Read the model definition and answer for the solid it produces. Units are mm, in the model's axes. Face numbers are marked on the shaded views. A direction names the side the tool comes from. Coordinates: 2 decimals unless noted, no trailing zeros. Write each loop counter-clockwise with the first axis right and the second up, starting at its lowest first coordinate (ties: lowest second). Pieces come first, ordered by that corner, then holes.
Item 1: Section D-D (z = -31) is taken. Give the vertices of the cut face in (x, y), then the cut area to 3 significant figures.
Item 2: A tool of negligible diameter and unlimited length cuts with its end or side. For the marked faces 1, 2, 3 and 4, from which of +Z, -Z, +X, -X, +Y, -Y can it reach the whole face along a straight path? Write none if from no direction.
Item 3: Straight lines are drawn through the part: probe 1 along Y at (x, z) = (-27, -81); probe 2 along Z at (x, y) = (-8.5, 10); probe 3 along Z at (x, y) = (-8.5, 41.5). For each, find the intervals that lie inside material, in ascending order.
Item 4: Section C-C (y = 25) is taken. Give the vertices of the cut face in (x, z).
Item 5: Each of these flat-tipped pins is pushed along its axis until it touches: P1, Ø1.5, axis at y = 23.5, z = -97.5, coming from the +X side; P2, Ø8, axis at x = -10, z = -58, coming from the +Y side; P3, Ø2, axis at x = -4.5, z = 14, coming from the -Y side. Where does it stop, or does it pass through?
Item 6: Section A-A (x = -8.5) is taken. Give the vertices of the cut face in (y, z).
Item 7: Determine the mould class of the marked faces 5, 6 and 7 for opening direction Z: released by +Z, released by -Z, zero draft, split by the parting line, or undercut.
Item 8: Section B-B (z = -81) is taken. Give the vertices of the cut face in (x, y), then the cut area to 3 significant figures.
Autodesk Inventor part; units mm, degrees
ref_plane "YZ Plane" through (0, 0, 0) normal (1, 0, 0) x (0, 1, 0)
ref_plane "XZ Plane" through (0, 0, 0) normal (0, 1, 0) x (-1, 0, 0)
ref_plane "XY Plane" through (0, 0, 0) normal (0, 0, 1) x (1, 0, 0)
sketch "Sketch1" plane through (0, 0, 0) normal (0, 1, 0) x (-1, 0, 0)
  arc A0 (35, -5) -> (0, 30) centre (0, -5) ccw
  line L0 (34.641, 0) -> (0, 0)
  line L1 (-35, -5) -> (-35, -100) construction
  line L2 (-35, -100) -> (0, -100) construction
  line L3 (35, -100) -> (35, -5)
  line L4 (0, -100) -> (0, 30)
  arc A1 (0, 30) -> (-35, -5) centre (0, -5) ccw construction
  line L5 (0, -5) -> (-35, -5) construction
  line L6 (0, -100) -> (35, -100)
  dimension "d0" = 70
  dimension "d1" = 130
  dimension "d32" = 30
  dimension "d33" = 35
  dimension "d34" = 5
extrude "Extrusion1" add sketch "Sketch1" along normal blind 50
sketch "Sketch2" plane through (0, 0, 30) normal (1, 0, 0) x (0, 0, -1)
  line L0 (19, 49) -> (27.5, 49)
  line L1 (59, 49) -> (59, 40)
  line L2 (59, 9) -> (19, 9)
  line L3 (19, 9) -> (19, 14)
  line L4 (19, 40) -> (12, 40)
  line L5 (12, 40) -> (12, 37)
  line L6 (12, 37) -> (19, 37)
  line L7 (19, 37) -> (19, 40) construction
  line L8 (19, 17) -> (14, 17)
  line L9 (14, 17) -> (14, 14)
  line L10 (14, 14) -> (19, 14)
  line L11 (19, 14) -> (19, 17) construction
  line L12 (59, 40) -> (66, 40)
  line L13 (66, 40) -> (66, 37)
  line L14 (66, 37) -> (59, 37)
  line L15 (59, 37) -> (59, 40) construction
  line L16 (27.5, 49) -> (32.5, 49) construction
  line L17 (32.5, 49) -> (32.5, 54)
  line L18 (32.5, 54) -> (27.5, 54)
  line L19 (27.5, 54) -> (27.5, 49)
  line L20 (0, 50) -> (130, 50)
  line L21 (19, 40) -> (19, 49)
  line L22 (19, 37) -> (19, 40) construction
  line L23 (19, 17) -> (19, 37)
  line L24 (19, 14) -> (19, 17) construction
  line L25 (59, 40) -> (59, 37) construction
  line L26 (59, 37) -> (59, 9)
  line L27 (27.5, 49) -> (32.5, 49) construction
  line L28 (32.5, 49) -> (59, 49)
  line L29 (9, 22) -> (19, 22)
  line L30 (19, 22) -> (19, 7)
  line L31 (19, 2) -> (9, 2)
  line L32 (9, 2) -> (9, 22)
  line L33 (19, 2) -> (76, 2)
  line L34 (19, 49) -> (19, 50)
  line L35 (59, 49) -> (59, 50)
  line L36 (71, 7) -> (71, 50)
  line L37 (71, 50) -> (76, 50)
  line L38 (76, 50) -> (76, 2)
  line L39 (71, 7) -> (19, 7)
  line L40 (0, 0) -> (0, 50)
  line L41 (30, 54) -> (30, 14.5)
  point P0 (66, 38.5)
  point P1 (19, 9)
  point P2 (32.5, 50)
  point P3 (27.5, 50)
  point P4 (19, 9)
  dimension "d5" = 3
  dimension "d6" = 3
  dimension "d7" = 5
  dimension "d8" = 40
  dimension "d9" = 5
  dimension "d10" = 5
  dimension "d11" = 36
  dimension "d12" = 40
  dimension "d13" = 7
  dimension "d14" = 5
  dimension "d15" = 7
  dimension "d16" = 9
  dimension "d18" = 1
  dimension "d20" = 10
  dimension "d21" = 5
  dimension "d22" = 20
  dimension "d26" = 5
  dimension "d27" = 5
  dimension "d28" = 57
  dimension "d29" = 48
  dimension "d30" = 5
  dimension "d36" = 30
extrude "Extrusion2" cut sketch "Sketch2" against normal blind 10 contours L34 L20 L19 L0 | L0 L19 L20 L17 L28 L1 L12 L13 L14 L26 L2 L3 L30 L23 L6 L5 L4 L21 | L20 L35 L28 L17 | L23 L8 L9 L10 L3 L30 L39 L36 L20 L38 L33 L31 L32 L29 | L30 L10 L9 L8
sketch "Sketch3" plane through (-35, 0, -100) normal (-1, 0, 0) x (0, 0, 1)
  circle A0 centre (19, 25) radius 35
  line L0 (130, 0) -> (130, 50)
  line L1 (54, 50) -> (54, 2)
  line L2 (19, 25) -> (130, 25)
  point P0 (100, 0)
  dimension "d37" = 70
extrude "Extrusion3" add sketch "Sketch3" against normal up to surface (35 mm away)
sketch "Sketch4" plane through (0, 0, 0) normal (0, -1, 0) x (1, 0, 0)
  arc A0 (0, 5) -> (0, -5) centre (0, 0) ccw
  line L0 (0, 5) -> (0, -5)
  line L1 (0, -46) -> (0, 21)
  dimension "d41" = 10
extrude "Extrusion4" add sketch "Sketch4" along normal blind 5
sketch "Sketch5" plane through (0, 0, 30) normal (1, 0, 0) x (0, 0, -1)
  arc A0 (86.5051, 0) -> (86.5051, 50) centre (111, 25) ccw
  circle A1 centre (111, 25) radius 35
  line L0 (76, 30) -> (111, 30)
  line L1 (111, 30) -> (111, 20)
  line L2 (111, 20) -> (76, 20)
  line L3 (76, 20) -> (76, 30)
  line L4 (76, 50) -> (76, 2)
  point P0 (30, 0)
  point P1 (86.5051, 0)
  point P2 (76, 25)
  point P3 (76.359, 20)
  point P4 (76.359, 30)
  dimension "d46" = 10
extrude "Extrusion5" cut sketch "Sketch5" against normal blind 22.5
sketch "Sketch6" plane through (-22.5, 0, 30) normal (1, 0, 0) x (0, 0, -1)
  arc A0 (86.5051, 0) -> (86.5051, 50) centre (111, 25) ccw
  circle A1 centre (111, 25) radius 12.5
  point P0 (30, 0)
  dimension "d47" = 25
extrude "Extrusion6" cut sketch "Sketch6" against normal blind 7
equation "\"d33\" = 0.5 * d0"
properties part number "wirst 2 right"
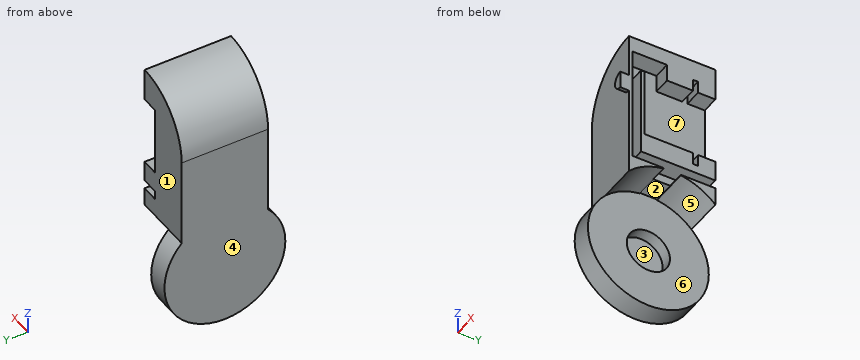
Established:
1. outline: (-35, 0) - (0, 0) - (0, 2) - (-10, 2) - (-10, 7) - (0, 7) - (0, 37) - (-10, 37) - (-10, 40) - (0, 40) - (0, 50) - (-35, 50) - close
1. area: 1,670 mm2
2. face 1: +Z, +X, -X, +Y
2. face 2: -Z, +X
2. face 3: +X
2. face 4: +Z, -Z, -X, +Y, -Y
3. probe 1: y = -10 to 12.5, 37.5 to 60
3. probe 2: z = -49.38 to -46, -41 to -29, 21 to 28.95
3. probe 3: z = -50.13 to -46, -41 to -29, 11 to 28.95
4. outline: (-35, -116) - (-22.5, -116) - (-22.5, -93.5) - (-29.5, -93.5) - (-29.5, -68.5) - (-22.5, -68.5) - (-22.5, -46) - (-10, -46) - (-10, -41) - (0, -41) - (0, -29) - (-10, -29) - (-10, 11) - (0, 11) - (0, 30) arc R35 ccw to (-35, -5) - close
5. P1: stops at x = -22.5
5. P2: stops at y = 50
5. P3: stops at y = 0
6. outline: (0, -56.51) arc R35 cw to (20, -46.36) - (20, -46) - (2, -46) - (2, 21) - (22, 21) - (22, 11) - (37, 11) - (37, 18) - (40, 18) - (40, 11) - (50, 11) - (50, 28.95) - (0, 28.95) - close; (7, -41) - (50, -41) - (50, -29) - (40, -29) - (40, -36) - (37, -36) - (37, -29) - (9, -29) - (9, 11) - (7, 11) - close; (30, -46.36) arc R35 cw to (50, -56.51) - (50, -46) - (30, -46) - close
7. face 5: released by -Z
7. face 6: zero draft
7. face 7: undercut
8. outline: (-35, -10) - (-22.5, -10) - (-22.5, 12.5) - (-29.5, 12.5) - (-29.5, 37.5) - (-22.5, 37.5) - (-22.5, 60) - (-35, 60) - close
8. area: 700 mm2
